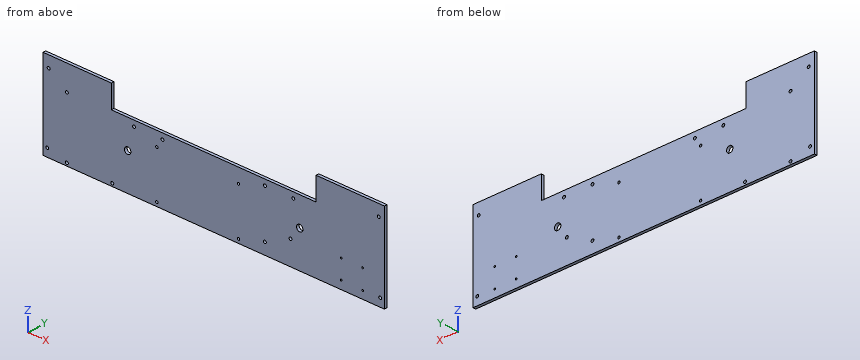
from build123d import *

# Parameters (mm, degrees)
BOSS_EXTRUDE1_DEPTH = 6.35
SKETCH3_R           = 3.302
SKETCH3_R_2         = 3.175
SKETCH3_R_3         = 7.14375
SKETCH3_R_4         = 1.905
CUT_EXTRUDE1_DEPTH  = 7.62
SKETCH5_R           = 2.667
SKETCH5_R_2         = 3.175
CUT_EXTRUDE2_DEPTH  = 7.62


with BuildPart() as part:
    # Sketch1 → Boss-Extrude1 (new body)
    with BuildSketch(Plane(origin=(0, 0, 0), x_dir=(1, 0, 0), z_dir=(0, 1, 0))):
        Polygon((0, 0), (457.2, 0), (457.2, -50.8), (609.6, -50.8), (609.6, 144.78), (-152.4, 144.78), (-152.4, -50.8), (0, -50.8), align=None)
    extrude(amount=BOSS_EXTRUDE1_DEPTH)

    # Sketch3 → Cut-Extrude1 (cut)
    with BuildSketch(Plane(origin=(0, 6.35, 0), x_dir=(1, 0, 0), z_dir=(0, 1, 0))):
        with Locations((-139.7, -25.4)):
            Circle(SKETCH3_R)
        with Locations((-99.1108, 5.0292)):
            Circle(SKETCH3_R_2)
        with Locations((-142.875, 126.81712)):
            Circle(SKETCH3_R)
        with Locations((-99.1108, 138.3792)):
            Circle(SKETCH3_R_2)
        with Locations((2.413, 138.3792)):
            Circle(SKETCH3_R_2)
        with Locations((36.576, 63.5)):
            Circle(SKETCH3_R_3)
        with Locations((600.075, 126.81712)):
            Circle(SKETCH3_R_2)
        with Locations((596.9, -25.4)):
            Circle(SKETCH3_R_2)
        with Locations((560.959, 127.8636)):
            Circle(SKETCH3_R_4)
        with Locations((513.207, 84.8106)):
            Circle(SKETCH3_R_4)
        with Locations((560.959, 84.8106)):
            Circle(SKETCH3_R_4)
        with Locations((513.207, 126.81712)):
            Circle(SKETCH3_R_4)
        with Locations((420.624, 63.5)):
            Circle(SKETCH3_R_3)
    extrude(amount=-CUT_EXTRUDE1_DEPTH, mode=Mode.SUBTRACT)

    # Sketch5 → Cut-Extrude2 (cut)
    with BuildSketch(Plane(origin=(0, 6.35, 0), x_dir=(1, 0, 0), z_dir=(0, 1, 0))):
        with Locations((101.6, 136.144)):
            Circle(SKETCH5_R)
        with Locations((101.6, 31.75)):
            Circle(SKETCH5_R)
        with Locations((400.05, 91.44)):
            Circle(SKETCH5_R_2)
        with Locations((406.4, 12.7)):
            Circle(SKETCH5_R_2)
        with Locations((342.9, 119.38)):
            Circle(SKETCH5_R_2)
        with Locations((342.9, 12.7)):
            Circle(SKETCH5_R_2)
        with Locations((283.8704, 136.144)):
            Circle(SKETCH5_R)
        with Locations((283.8704, 31.75)):
            Circle(SKETCH5_R)
        with Locations((114.3, 12.7)):
            Circle(SKETCH5_R_2)
        with Locations((50.8, 12.7)):
            Circle(SKETCH5_R_2)
    extrude(amount=-CUT_EXTRUDE2_DEPTH, mode=Mode.SUBTRACT)


solid = part.part
Here's how the part is built. I have some questions about the finished solid (model axes, mm). Round coordinates to 2 decimals unless told otherwise and drop trailing zeros. Loops run counter-clockwise (first coordinate to the right, second up) from the corner with the lowest first, then second, coordinate; pieces in that order, holes last.
1. If we section it at A-A on z = -63.5: Write out the boundary of the cut face in (x, y), plus the area to 3 significant figures.
Answer list:
outline: (-152.4, 0) - (29.43, 0) - (29.43, 6.35) - (-152.4, 6.35) - close; (43.72, 0) - (413.48, 0) - (413.48, 6.35) - (43.72, 6.35) - close; (427.77, 0) - (609.6, 0) - (609.6, 6.35) - (427.77, 6.35) - close
area: 4,660 mm2
2. If I drill on line 1 along X through (y, z) = (1.5, 25.4) (3 decimals); line 2 along X through (y, z) = (1.5, -12.7) (3 decimals); line 3 along Z through (x, y) = (342.9, 1.75) (3 decimals), over which ranges is the centre line in solid material (lowest first)?
Answer list:
line 1: x = -152.4 to -143.002, -136.398 to 0, 457.2 to 593.725, 600.075 to 609.6
line 2: x = -152.4 to 47.625, 53.975 to 111.125, 117.475 to 339.725, 346.075 to 403.225, 409.575 to 609.6
line 3: z = -144.78 to -122.555, -116.205 to -15.875, -9.525 to 0
3. If we section it at B-B on y = 2: Count the separate pieces of the cut face and the enclosed holes in it, plus the area to 3 significant figures.
Answer list:
separate pieces: 1
enclosed holes: 23
area: 125,000 mm2
4. If we section it at C-C on x = 242.5: Write out the boundary of the cut face in (y, z), plus the area to 3 significant figures.
Answer list:
outline: (0, -144.78) - (6.35, -144.78) - (6.35, 0) - (0, 0) - close
area: 919 mm2
5. For P1, Ø4.5, axis at x = 101.6, z = -136.144, coming from the +Y side; P2, Ø10, axis at x = -99.11, z = -138.38, coming from the +Y side, each with a flat end and sliding along its axis, tell me the tip position at first contact or that it passes through.
Answer list:
P1: passes through
P2: stops at y = 6.35
